Geometry: final body of the model. Coordinates: model frame, mm. Coordinates: 2 decimals unless noted, no trailing zeros. Order: outer loops, then holes, each group sorted by start corner. A loop starts at its lowest first (then second) coordinate and runs counter-clockwise, first axis right, second up. Notation, with made-up numbers: M -36.5,27 L -19.5,27 A14 cw -19.5,50 Z; hole C 12,88.5 d11. An arc over 180 degrees is marked long. Use CSV: the item, a comma, the result in double quotes. Start each with the question number.
1. Section query A-A on y = 0. Return the cut outline in (x, z), and give its area (3 significant figures).
2. First-contact query: P1, Ø1, axis at y = -1, z = 0.5, coming from the +X side. Flat tip, straight axial feed; report the tip coordinate or a pass-through.
3. Pull-direction query (Y, two-part tool) for faces 1 (the cylindrical face through (-12, 0, 1)), 2 (the cylindrical face through (0, 1, 1)), 3 (the cylindrical face through (-10.8, 0.6, 1)), 4 (the flat face through (-5, 2, 1)); classes: pulls with the +Y half, pulls with the -Y half, needs draft (parallel to the pull), parting line crosses it, or undercut.
4. Material intervals for line 1 (X direction, y = 0.05, z = 0.3); line 2 (Y direction, x = 0, z = 0.9); line 3 (X direction, y = -0.9, z = 1.75), sorted ascending.
5. Section query B-B on z = 1.35. Return the cut outline in (x, y), and give its area (3 significant figures).
6. Section query D-D on y = -1.5. Return the cut outline in (x, z), and give its area (3 significant figures).
7. Section query C-C on y = -0.6. Return the cut outline in (x, z).
Autodesk Inventor part; units mm, degrees
ref_plane "YZ Plane" through (0, 0, 0) normal (1, 0, 0) x (0, 1, 0)
ref_plane "XZ Plane" through (0, 0, 0) normal (0, 1, 0) x (-1, 0, 0)
ref_plane "XY Plane" through (0, 0, 0) normal (0, 0, 1) x (1, 0, 0)
sketch "Sketch1" plane through (0, 0, 0) normal (0, 0, 1) x (1, 0, 0)
  circle A0 centre (0, 0) radius 1
  circle A1 centre (-10, 0) radius 1
  line L0 (-10, 2) -> (0, 2)
  arc A2 (0, -2) -> (0, 2) centre (0, 0) ccw
  line L1 (0, -2) -> (-10, -2)
  arc A3 (-10, 2) -> (-10, -2) centre (-10, 0) ccw
  dimension "d0" = 2
  dimension "d1" = 10
  dimension "d2" = 2
extrude "Extrusion1" add sketch "Sketch1" along normal blind 2
properties part number "panto_linkageA"
Results list:
1,outline,"M -12,0 L -11,0 L -11,2 L -12,2 Z; M -9,0 L -1,0 L -1,2 L -9,2 Z; M 1,0 L 2,0 L 2,2 L 1,2 Z"
1,area,"20.0 mm²"
2,P1,"stops at x = 1.94"
3,face 1,"parting line crosses it"
3,face 2,"undercut"
3,face 3,"undercut"
3,face 4,"pulls with the +Y half"
4,line 1,"x = -12 to -11, -9 to -1, 1 to 2"
4,line 2,"y = -2 to -1, 1 to 2"
4,line 3,"x = -11.79 to -10.44, -9.56 to -0.44, 0.44 to 1.79"
5,outline,"M -10,-2 L 0,-2 A2 ccw 0,2 L -10,2 A2 ccw Z; hole C -10,0 d2; hole C 0,0 d2"
5,area,"46.3 mm²"
6,outline,"M -11.32,0 L 1.32,0 L 1.32,2 L -11.32,2 Z"
6,area,"25.3 mm²"
7,outline,"M -11.91,0 L -10.8,0 L -10.8,2 L -11.91,2 Z; M -9.2,0 L -0.8,0 L -0.8,2 L -9.2,2 Z; M 0.8,0 L 1.91,0 L 1.91,2 L 0.8,2 Z"
